Here's how the part is built. I have some questions about the finished solid (model axes, mm). A direction names the side the tool comes from. Round coordinates to 2 decimals unless told otherwise and drop trailing zeros. Order: outer loops, then holes, each group sorted by start corner. A loop starts at its lowest first (then second) coordinate and runs counter-clockwise, first axis right, second up. Notation, with made-up numbers: (79.5, 75) - (94.5, 75) arc R16 ccw to (94.5, 88) - close; hole circle Ø4 at (-40, 48.25). An arc over 180 degrees is marked (long way). One line per item, written item: value.
from build123d import *

# Parameters (mm, degrees)
BOSS_EXTRUDE1_DEPTH  = 1
CUT_EXTRUDE1_DEPTH   = 1.25
BOSS_EXTRUDE2_DEPTH  = 1
FILLET1_R            = 0.5
FILLET2_R            = 0.5
SKETCH5_W            = 8
SKETCH5_H            = 5
BOSS_EXTRUDE3_DEPTH  = 1.25
FILLET3_R            = 0.5
FILLET1_OF_MIRROR6_R = 0.5
FILLET4_R            = 0.5
SKETCH6_R            = 1.15
CUT_EXTRUDE2_DEPTH   = 29.120631136


with BuildPart() as part:
    # Sketch2 → Boss-Extrude1 (new body)
    with BuildSketch(Plane(origin=(0, 0, 0), x_dir=(1, 0, 0), z_dir=(0, 1, 0))):
        with BuildLine():
            Line((15, -10), (-9.633249581, -10))
            ThreePointArc((-9.633249581, -10), (-15, 0), (-9.633249581, 10))
            Line((-9.633249581, 10), (15, 10))
            Line((15, 10), (15, -10))
        make_face()
    extrude(amount=BOSS_EXTRUDE1_DEPTH)

    # Sketch3 → Cut-Extrude1 (cut)
    with BuildSketch(Plane(origin=(0, 1, 0), x_dir=(1, 0, 0), z_dir=(0, 1, 0))):
        with BuildLine():
            Line((-8, 4.8), (-2, 4.8))
            Line((-2, 4.8), (-2, -4.8))
            Line((-2, -4.8), (-8, -4.8))
            ThreePointArc((-8, -4.8), (-12.8, 0), (-8, 4.8))
        make_face()
    extrude(amount=-CUT_EXTRUDE1_DEPTH, mode=Mode.SUBTRACT)

    # Sketch4 → Boss-Extrude2 (add)
    with BuildSketch(Plane(origin=(0, 1, 0), x_dir=(1, 0, 0), z_dir=(0, 1, 0))):
        Polygon((9, 10), (9, 17), (15, 10), align=None)
    boss_extrude2 = extrude(amount=-BOSS_EXTRUDE2_DEPTH)

    # Fillet1
    fillet1_edges = [part.edges().sort_by_distance(p)[0] for p in [
        (9, 0.5, -17),
    ]]
    fillet(fillet1_edges, radius=FILLET1_R)

    # Fillet2
    fillet2_edges = [part.edges().sort_by_distance(p)[0] for p in [
        (9, 0.5, -10),
    ]]
    fillet(fillet2_edges, radius=FILLET2_R)

    # Sketch5 → Boss-Extrude3 (add)
    with BuildSketch(Plane(origin=(0, 1, 0), x_dir=(1, 0, 0), z_dir=(0, 1, 0))):
        with Locations((19, 6)):
            Rectangle(SKETCH5_W, SKETCH5_H)
    boss_extrude3 = extrude(amount=-BOSS_EXTRUDE3_DEPTH)

    # Fillet3
    fillet3_edges = [part.edges().sort_by_distance(p)[0] for p in [
        (15, 0.5, -3.5),
        (15, 0.5, -8.5),
        (15, 0.5, -10),
    ]]
    fillet(fillet3_edges, radius=FILLET3_R)

    # Mirror6: Boss-Extrude2, Boss-Extrude3 across plane
    add(boss_extrude2.mirror(Plane.XY))
    add(boss_extrude3.mirror(Plane.XY))

    # Fillet1 of Mirror6
    fillet1_of_mirror6_edges = [part.edges().sort_by_distance(p)[0] for p in [
        (9, 0.5, 17),
    ]]
    fillet(fillet1_of_mirror6_edges, radius=FILLET1_OF_MIRROR6_R)

    # Fillet4
    fillet4_edges = [part.edges().sort_by_distance(p)[0] for p in [
        (9, 0.5, 10),
        (15, 0.5, 8.5),
        (15, 0.5, 3.5),
        (15, 0.5, 10),
    ]]
    fillet(fillet4_edges, radius=FILLET4_R)

    # Sketch6 → Cut-Extrude2 (cut, through all)
    with BuildSketch(Plane.XZ):
        with Locations(Location((-5, -7.5, 0), (0, 0, 270))):
            Circle(SKETCH6_R)
        with Locations(Location((11, -6, 0), (0, 0, 270))):
            Circle(SKETCH6_R)
        with Locations(Location((11, 6, 0), (0, 0, 270))):
            Circle(SKETCH6_R)
        with Locations(Location((-5, 7.5, 0), (0, 0, 270))):
            Circle(SKETCH6_R)
    extrude(amount=-CUT_EXTRUDE2_DEPTH, mode=Mode.SUBTRACT)


solid = part.part
Q1. If we section it at A-A, the plane z = 0: Please give me the cut outline in (x, y).
Results list:
outline: (-15, 0) - (-12.8, 0) - (-12.8, 1) - (-15, 1) - close; (-2, 0) - (15, 0) - (15, 1) - (-2, 1) - close
Q2. If we section it at D-D, the plane x = -10.5: Please give me the cut outline in (y, z).
Results list:
outline: (0, -9.37) - (1, -9.37) - (1, -4.1) - (0, -4.1) - close; (0, 4.1) - (1, 4.1) - (1, 9.37) - (0, 9.37) - close
Q3. Which directions (+Z, -Z, +X, -X, +Y, -Y) give clear straight access to the entire face, cutting with the end or side of a thin tool? Please do faces 4 (the flat face through (9, 0.5, -13)), 5 (the cylindrical face through (-15, 0.5, 0.2)), 6 (the flat face through (-0.4, 0.5, 10)), 7 (the flat face through (15, 0.5, 9.4)), 8 (the flat face through (-2, 0.5, -0.1)).
Results list:
face 4: -Z, -X, +Y, -Y
face 5: -X, +Y, -Y
face 6: +Z, -X, +Y, -Y
face 7: +Z, +X, +Y, -Y
face 8: +Y, -Y
Q4. We'd pull the mould along Z, two halves only. Please class faces 1 (the cylindrical face through (-4.03, 0.49, -8.12)), 2 (the flat face through (12.345, 0.507, 13.098)), 3 (the cylindrical face through (9.319, 0.493, -16.114)): released by +Z, released by -Z, zero draft, split by the parting line, or undercut.
Results list:
face 1: undercut
face 2: released by +Z
face 3: released by -Z
Q5. If we section it at C-C, the plane y = 0.6: Give the number of separate pieces and of enclosed holes in the cut face, then the cut area to 3 significant figures.
Results list:
separate pieces: 1
enclosed holes: 5
area: 579 mm²
Q6. If we section it at B-B, the plane x = -5: Please give me the cut outline in (y, z).
Results list:
outline: (0, -10) - (1, -10) - (1, -8.65) - (0, -8.65) - close; (0, -6.35) - (1, -6.35) - (1, -4.8) - (0, -4.8) - close; (0, 4.8) - (1, 4.8) - (1, 6.35) - (0, 6.35) - close; (0, 8.65) - (1, 8.65) - (1, 10) - (0, 10) - close
Q7. Will these pins go through, and if not, where does the flat tip stop? pin 1 (0.5 mm diameter, centred on y = 0.5, z = 0.5, fed in from +X); pin 2 (10 mm diameter, centred on x = -7, z = 6.5, fed in from -Y); pin 3 (1.4 mm diameter, centred on x = -5, z = 7.5, fed in from -Y).
Results list:
pin 1: x = 15
pin 2: y = 0
pin 3: through
Q8. If I drill on line 1 along Z through (x, y) = (21.5, 0.1); line 2 along Z through (x, y) = (12, 0.8); line 3 along X through (y, z) = (0.6, -7), over which ranges is the centre line in solid material (lowest first)?
Results list:
line 1: -8.5 to -3.5, 3.5 to 8.5
line 2: -13.5 to -6.57, -5.43 to 5.43, 6.57 to 13.5
line 3: -12.75 to -6.04, -3.96 to 10.43, 11.57 to 23
